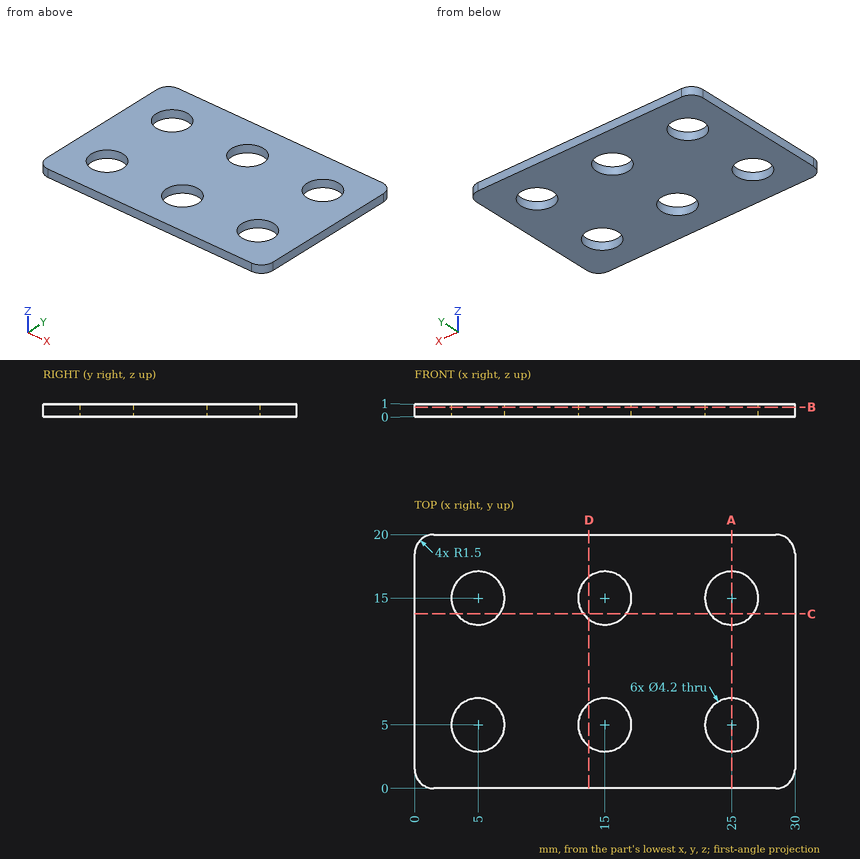
The figure shows three views and two pictorial views of one solid part (mm, origin at its lowest corner). Answer the questions. Round coordinates to 2 decimals unless told otherwise and drop trailing zeros. Loops run counter-clockwise (first coordinate to the right, second up) from the corner with the lowest first, then second, coordinate; pieces in that order, holes last. Notation, with made-up numbers: M 53.25,87.5 L 64.25,87.5 A30 cw 64.25,126.5 Z; hole C 81.5,-19.75 d7. An arc over 180 degrees is marked long. Write each question's results on one line, items separated by ' | '. Start each with the question number.
1) Find section C-C on y = 13.75. Write down the section's boundary in (x, z).
2) Find section A-A on x = 25. Write down the section's boundary in (y, z).
3) Each of these flat-tipped pins is pushed along its axis until it touches: pin 1 (3.5 mm diameter, centred on x = 15, y = 5, fed in from +Z); pin 2 (5.5 mm diameter, centred on x = 15, y = 15, fed in from +Z). Where does it stop, or does it pass through?
4) Find section B-B on z = 0.75. Write down the section's boundary in (x, y).
5) Find section D-D on x = 13.75. Write down the section's boundary in (y, z).
6) Straight lines are drawn through the part: probe 1 along Y at (x, z) = (5, 0.7); probe 2 along X at (y, z) = (6, 0.7); probe 3 along X at (y, z) = (13.5, 0.95). For each, find the intervals that lie inside material, in ascending order.
Final values:
1) outline: M 0,0 L 3.31,0 L 3.31,1 L 0,1 Z; M 6.69,0 L 13.31,0 L 13.31,1 L 6.69,1 Z; M 16.69,0 L 23.31,0 L 23.31,1 L 16.69,1 Z; M 26.69,0 L 30,0 L 30,1 L 26.69,1 Z
2) outline: M 0,0 L 2.9,0 L 2.9,1 L 0,1 Z; M 7.1,0 L 12.9,0 L 12.9,1 L 7.1,1 Z; M 17.1,0 L 20,0 L 20,1 L 17.1,1 Z
3) pin 1: through | pin 2: z = 1
4) outline: M 0,1.5 A1.5 ccw 1.5,0 L 28.5,0 A1.5 ccw 30,1.5 L 30,18.5 A1.5 ccw 28.5,20 L 1.5,20 A1.5 ccw 0,18.5 Z; hole C 5,5 d4.2; hole C 5,15 d4.2; hole C 15,5 d4.2; hole C 15,15 d4.2; hole C 25,5 d4.2; hole C 25,15 d4.2
5) outline: M 0,0 L 3.31,0 L 3.31,1 L 0,1 Z; M 6.69,0 L 13.31,0 L 13.31,1 L 6.69,1 Z; M 16.69,0 L 20,0 L 20,1 L 16.69,1 Z
6) probe 1: 0 to 2.9, 7.1 to 12.9, 17.1 to 20 | probe 2: 0 to 3.15, 6.85 to 13.15, 16.85 to 23.15, 26.85 to 30 | probe 3: 0 to 3.53, 6.47 to 13.53, 16.47 to 23.53, 26.47 to 30
